```python
from build123d import *

# Parameters (mm, degrees)
SKETCH1_R           = 8.334375
BOSS_EXTRUDE1_DEPTH = 2.54
SKETCH3_R           = 3.175
BOSS_EXTRUDE2_DEPTH = 6.35
CIRPATTERN1_COUNT   = 3


with BuildPart() as part:
    # Sketch1 → Boss-Extrude1 (new body)
    with BuildSketch(Plane(origin=(0, 0, 0), x_dir=(1, 0, 0), z_dir=(0, 1, 0))):
        with BuildLine():
            Line((2.54, 11.225600781), (2.54, 36.195))
            ThreePointArc((2.54, 36.195), (0, 41.275), (-2.54, 36.195))
            Line((-2.54, 36.195), (-2.54, 11.225600781))
            ThreePointArc((-2.54, 11.225600781), (0, -11.509375), (2.54, 11.225600781))
        make_face()
        with Locations(Location((0, 0, 0), (0, 0, 270))):
            Circle(SKETCH1_R, mode=Mode.SUBTRACT)
    boss_extrude1 = extrude(amount=BOSS_EXTRUDE1_DEPTH)

    # Sketch3 → Boss-Extrude2 (add)
    with BuildSketch(Plane(origin=(0, 2.54, 0), x_dir=(1, 0, 0), z_dir=(0, 1, 0))):
        with Locations(Location((0, 38.1, 0), (0, 0, 216.869897646))):
            Circle(SKETCH3_R)
    boss_extrude2 = extrude(amount=BOSS_EXTRUDE2_DEPTH)

    # CirPattern1: Boss-Extrude1, Boss-Extrude2 ×3 about axis
    cirpattern1_axis = Axis((0, 0, 0), (0, 1, 0))
    add([boss_extrude1.rotate(cirpattern1_axis, i * 360 / CIRPATTERN1_COUNT) for i in range(1, CIRPATTERN1_COUNT)])
    add([boss_extrude2.rotate(cirpattern1_axis, i * 360 / CIRPATTERN1_COUNT) for i in range(1, CIRPATTERN1_COUNT)])


solid = part.part
```
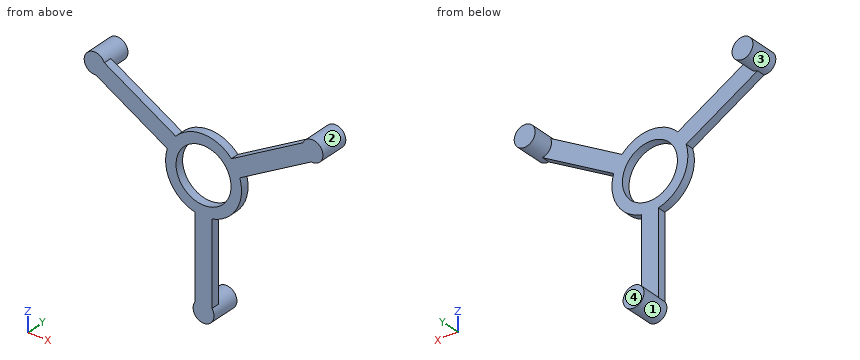
Geometry check sheet. Reference: the model listing, model coordinates, mm. Face numbers are marked on the shaded views. Give positions to 0.01 mm unless a question says otherwise; leave off trailing zeros. Loops run counter-clockwise (first coordinate to the right, second up) from the corner with the lowest first, then second, coordinate; pieces in that order, holes last. Notation, with made-up numbers: (37, 51) - (77, 51) arc R24 cw to (77, 86) - close; hole circle Ø7 at (2.5, 50). An arc over 180 degrees is marked (long way). Use CSV: the item, a comma, the result in double quotes. Start each with the question number.
Q1. Section check D-D, the plane y = 8. Record the cut outline in (x, z) (3 decimals), and give its area (3 significant figures).
Q2. Section check C-C, the plane x = 0. Record the cut outline in (y, z) (3 decimals), and give its area (3 significant figures).
Q3. Section check B-B, the plane z = 0. Record the cut outline in (x, y).
Q4. Scan lines: probe 1 along Z at (x, y) = (0, 1.6) (3 decimals); probe 2 along X at (y, z) = (6, -38); probe 3 along X at (y, z) = (1.1, 0). Record each from-to range of solid material in increasing order. Write a range as from..to.
Q5. Go/stop test with flat-tipped pins: pin 1 Ø5 at (y, z) = (2.5, 1) entering from -X; pin 2 Ø2 at (y, z) = (2, -20) entering from -X; pin 3 Ø0.8 at (y, z) = (1, -23) entering from +X. Record where each tip stops, or that it passes through.
Q6. Release check for a two-part mould opening along X. For the marked faces 1, 2, 3 and 4 record: +X half, -X half, draft (parallel to the pull), parting line (faces both ways), or undercut.
Findings below:
1,outline,"circle Ø6.35 at (-32.996, 19.05); circle Ø6.35 at (0, -38.1); circle Ø6.35 at (32.996, 19.05)"
1,area,"95.0 mm^2"
2,outline,"(0, -41.275) - (8.89, -41.275) - (8.89, -34.925) - (2.54, -34.925) - (2.54, -8.334) - (0, -8.334) - close; (0, 8.334) - (2.54, 8.334) - (2.54, 11.509) - (0, 11.509) - close"
2,area,"132 mm^2"
3,outline,"(-11.51, 0) - (-8.33, 0) - (-8.33, 2.54) - (-11.51, 2.54) - close; (8.33, 0) - (11.51, 0) - (11.51, 2.54) - (8.33, 2.54) - close"
4,probe 1,"z = -41.275..-8.334, 8.334..11.509"
4,probe 2,"x = -3.17..3.17"
4,probe 3,"x = -11.51..-8.33, 8.33..11.51"
5,pin 1,"stops at x = -11.51"
5,pin 2,"stops at x = -2.54"
5,pin 3,"stops at x = 2.54"
6,face 1,"parting line"
6,face 2,"undercut"
6,face 3,"undercut"
6,face 4,"draft"
